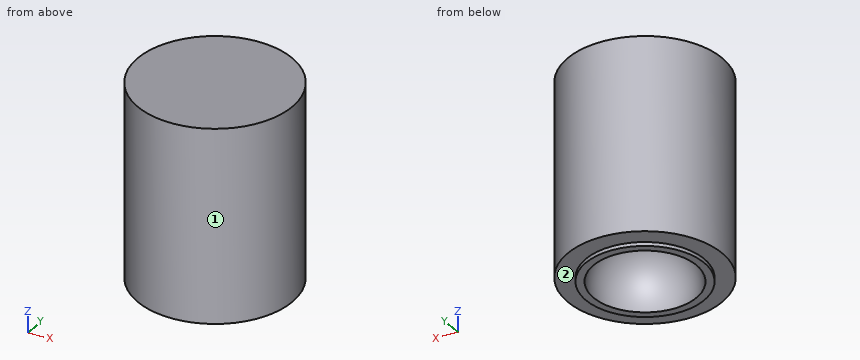
from build123d import *

# Parameters (mm, degrees)
F0_R     = 60
F1_DEPTH = 150
F2_R     = 46
F3_DEPTH = 3


# Not quite as in the source:
# - a feature names something its author has since deleted; it is built from what else it names


with BuildPart() as f1:
    # F0 (on Top) → F1 (new body)
    with BuildSketch(Plane.XY):
        Circle(F0_R)
    extrude(amount=F1_DEPTH)

    # F2 (on face) → F3 (join)
    with BuildSketch(Plane(origin=(0, 0, 0), x_dir=(1, 0, 0), z_dir=(0, 0, -1))):
        Circle(F2_R)
    extrude(amount=F3_DEPTH)

    # F4 (on face) → F5 (revolve, cut)
    with BuildSketch(Plane(origin=(0, 0, -3), x_dir=(1, 0, 0), z_dir=(0, 0, -1))):
        with BuildLine():
            Line((0, 40), (0, -40))
            ThreePointArc((0, -40), (40, 0), (0, 40))
        make_face()
    revolve(axis=Axis((0, 0, -3), (0, -1, 0)), mode=Mode.SUBTRACT)


solid = f1.part
For this review, take the finished solid that the model builds, in its own axes (mm). Face numbers are marked on the shaded views. A direction names the side the tool comes from. Round coordinates to 2 decimals unless told otherwise and drop trailing zeros. Order: outer loops, then holes, each group sorted by start corner. A loop starts at its lowest first (then second) coordinate and runs counter-clockwise, first axis right, second up. Notation, with made-up numbers: M 79,-4.5 L 122,-4.5 A14 ccw 122,1.5 Z; hole C 9,49.25 d10. An arc over 180 degrees is marked long. Use a Markdown table: item, result. Add a question column.
Item 1: Insertion check: pin 1 (1 mm diameter, centred on y = 38, z = 73.5, fed in from +X); pin 2 (3 mm diameter, centred on x = 33, y = -5.5, fed in from -Z); pin 3 (1.5 mm diameter, centred on x = -32.5, z = 120, fed in from +Y). Each pin has a flat end and moves straight along its axis. Give the tip position at first contact, or say it passes through.
Item 2: Add section D-D, the plane x = -42. Give the boundary of the cut face in (y, z).
Item 3: Add section C-C, the plane z = 16.5. Give the boundary of the cut face in (x, y).
Item 4: To check wall thickness, follow line 1 along Y through (x, z) = (2, 144); line 2 along Z through (x, y) = (-33.5, 44); line 3 along X through (y, z) = (-9.5, 5). State the ranges of each line that lie inside material, in increasing order.
Item 5: Tool access review of the marked faces 1 and 2: name each direction out of +Z, -Z, +X, -X, +Y, -Y from which nothing blocks a thin tool from reaching the whole face with its end or side.
Item 6: Add section A-A, the plane y = 0. Give the boundary of the cut face in (x, z).
Geometry results:
| question | item | result |
|---|---|---|
| 1 | pin 1 | stops at x = 46.84 |
| 1 | pin 2 | stops at z = 16.45 |
| 1 | pin 3 | stops at y = 50.91 |
| 2 | outline | M -42.85,0 L -18.76,0 L -18.76,-3 L 18.76,-3 L 18.76,0 L 42.85,0 L 42.85,150 L -42.85,150 Z |
| 3 | outline | C 0,0 d120; hole C 0,0 d69.85 |
| 4 | line 1 | y = -59.97 to 59.97 |
| 4 | line 2 | z = 0 to 150 |
| 4 | line 3 | x = -59.24 to -38.02, 38.02 to 59.24 |
| 5 | face 1 | +Z, -Z |
| 5 | face 2 | -Z |
| 6 | outline | M -60,0 L -46,0 L -46,-3 L -40,-3 A40 cw 40,-3 L 46,-3 L 46,0 L 60,0 L 60,150 L -60,150 Z |
